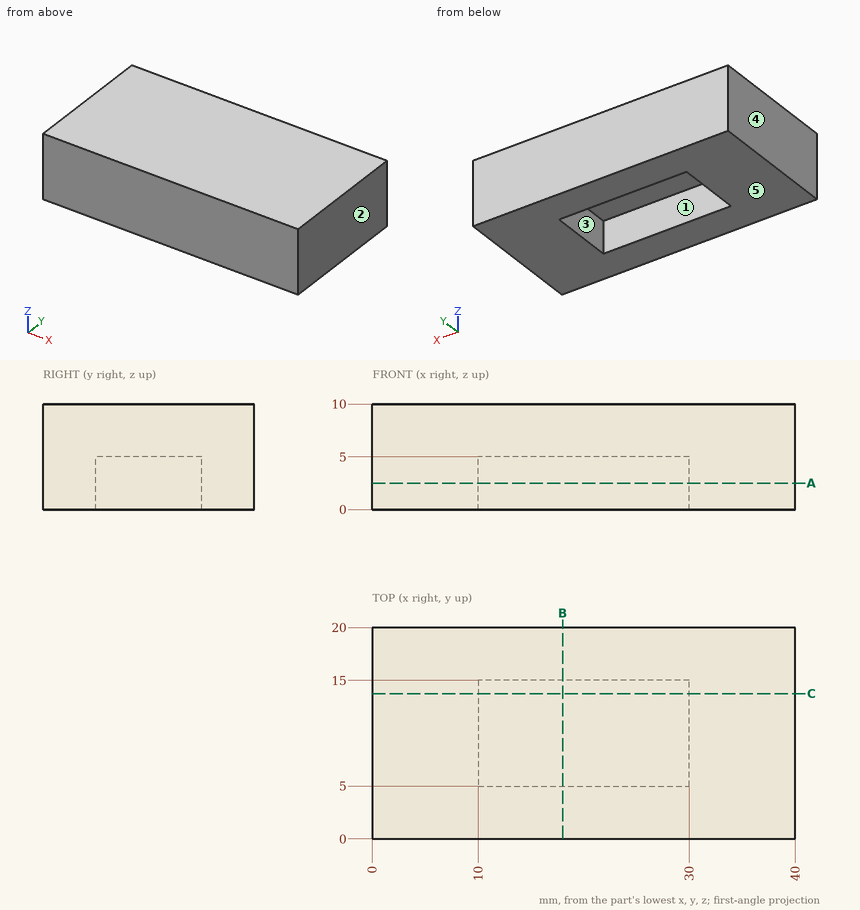
Job drawing, mm, ordinate dimensions from the low corner. One solid piece. A direction names the side the tool comes from. Round coordinates to 2 decimals unless told otherwise and drop trailing zeros. Loops run counter-clockwise (first coordinate to the right, second up) from the corner with the lowest first, then second, coordinate; pieces in that order, holes last. Notation, with made-up numbers: (41, -9.75) -> (56, -9.75) arc R34 ccw to (56, 20.25) -> close; hole circle Ø1 at (57, -32.75). An arc over 180 degrees is marked (long way). Use a Markdown table: item, result.
1) Pull direction X, two halves, no side cores. Call the marked faces 3, 4 and 5: pulls with the +X half, pulls with the -X half, needs draft (parallel to the pull), parting line crosses it, or undercut.
The answers:
| item | result |
|---|---|
| face 3 | undercut |
| face 4 | pulls with the -X half |
| face 5 | needs draft |
2) Tool access for the marked faces 1 and 2: list every direction of +Z, -Z, +X, -X, +Y, -Y with a clear straight run to the whole face (end or side of a thin tool).
The answers:
| item | result |
|---|---|
| face 1 | -Z |
| face 2 | +Z, -Z, +X, +Y, -Y |
3) Cut at A-A, the plane z = 2.5. List the corners of the cut face in (x, y), and give its area (3 significant figures).
The answers:
| item | result |
|---|---|
| outline | (0, 0) -> (40, 0) -> (40, 20) -> (0, 20) -> close; hole (10, 5) -> (30, 5) -> (30, 15) -> (10, 15) -> close |
| area | 600 mm2 |
4) Cut at C-C, the plane y = 13.75. List the corners of the cut face in (x, z), and give its area (3 significant figures).
The answers:
| item | result |
|---|---|
| outline | (0, 0) -> (10, 0) -> (10, 5) -> (30, 5) -> (30, 0) -> (40, 0) -> (40, 10) -> (0, 10) -> close |
| area | 300 mm2 |
5) Drop a flat-ended pin along its axis: pin 1 Ø1 at (x, y) = (16, 12) entering from -Z. Give the stop position or say it passes through.
The answers:
| item | result |
|---|---|
| pin 1 | stops at z = 5 |
6) Cut at B-B, the plane x = 18. List the corners of the cut face in (y, z).
The answers:
| item | result |
|---|---|
| outline | (0, 0) -> (5, 0) -> (5, 5) -> (15, 5) -> (15, 0) -> (20, 0) -> (20, 10) -> (0, 10) -> close |
7) Probe line 1 (X direction, y = 8.5, z = 0.5); line 2 (Y direction, x = 19.5, z = 3.75); line 3 (Z direction, x = 25, y = 14.5). List the from-to ranges inside material, lowest first. Write a range as [from, to].
The answers:
| item | result |
|---|---|
| line 1 | x = [0, 10], [30, 40] |
| line 2 | y = [0, 5], [15, 20] |
| line 3 | z = [5, 10] |
